Autodesk Inventor part; units mm, degrees
ref_plane "YZ Plane" through (0, 0, 0) normal (1, 0, 0) x (0, 1, 0)
ref_plane "XZ Plane" through (0, 0, 0) normal (0, 1, 0) x (-1, 0, 0)
ref_plane "XY Plane" through (0, 0, 0) normal (0, 0, 1) x (1, 0, 0)
sketch "Sketch1" plane through (0, 0, 0) normal (0, 1, 0) x (-1, 0, 0)
  line L0 (0, 0) -> (56, 0)
  line L1 (56, 0) -> (54.5, 0)
  line L2 (56, 0) -> (21.359, -20)
  line L3 (56, 0) -> (96, 0) construction
  line L4 (28, 0) -> (28, 5.9969)
  line L5 (0, 0) -> (34.641, -20)
  line L6 (28, 0) -> (28, -6)
  line L7 (28, -6) -> (78, -6)
  line L8 (28, -6) -> (-22, -6)
  line L9 (56, 0) -> (53.4019, -1.5)
  line L10 (53.4019, -1.5) -> (39.2598, -15.6421)
  line L11 (53.4019, -1.5) -> (73.4019, -1.5) construction
  line L12 (2.5981, -1.5) -> (16.7402, -15.6421)
  point P0 (48.9019, -6)
  point P1 (7.0981, -6)
  dimension "d0" = 56
  dimension "d3" = 40
  dimension "d4" = 150
  dimension "d5" = 6
  dimension "d6" = 50
  dimension "d7" = 50
  dimension "d8" = 3
  dimension "d9" = 20
  dimension "d10" = 135
extrude "Extrusion1" add sketch "Sketch1" along normal blind 6 contours L0 L6 L8 L5 | L0 L2 L7 L6 | L5 L8 L12 | L2 L10 L7
chamfer "Chamfer1" distance 2 angle 45 6 edges at (-48.9019, 3, -6) (-51.1519, 6, -3.75) (-51.1519, 0, -3.75) (-4.8481, 0, -3.75) (-7.0981, 3, -6) (-4.8481, 6, -3.75)
chamfer "Chamfer2" distance 2 angle 45 2 edges at (-37.0367, 0, -6) (-37.0367, 6, -6)
sketch "Sketch3" plane through (0, 0, 0) normal (0, -1, 0) x (1, 0, 0)
  line L0 (-49.0718, -4) -> (-56, 0)
  line L1 (-56, 0) -> (-32.5, 0)
  line L2 (-56, 0) -> (0, 0)
  line L3 (-32.5, 0) -> (-32.5, -2.5)
  line L4 (-6.9282, -4) -> (-49.0718, -4)
  circle A0 centre (-32.5, -2.5) radius 1.1
  dimension "d25" = 23.5
  dimension "d26" = 2.5
  dimension "d27" = 2.2
extrude "Extrusion3" cut sketch "Sketch3" against normal blind 50
properties part number "parallel_bar_long_hole_v1"
Check sheet for the modelled part. Datum: model origin and axes. Units: mm. A direction names the side the tool comes from. Round coordinates to 2 decimals unless told otherwise and drop trailing zeros. Loops run counter-clockwise (first coordinate to the right, second up) from the corner with the lowest first, then second, coordinate; pieces in that order, holes last. Notation, with made-up numbers: (27.5, 13.5) - (56.5, 13.5) arc R31 ccw to (56.5, 40.5) - close; hole circle Ø1 at (83, -23.75). An arc over 180 degrees is marked (long way). Write item = value, one per line. Start each with the question number.
Q1. Depth check by flat-ended pin: P1, Ø3, axis at y = 2, z = -5, coming from the +X side; P2, Ø1.3, axis at x = -32.5, z = -2.5, coming from the -Y side; P3, Ø1, axis at y = 1, z = -3, coming from the +X side. Enter the tip coordinate at first touch or a pass-through.
Q2. Release check for a two-part mould opening along X. For faces 1 (the face through (-28, 0, -2)), 2 (the face through (-31.45, 2.96, -2.17)), 3 (the face through (-2.094, 2.958, -1.209)) record: pulls with the +X half, pulls with the -X half, needs draft (parallel to the pull), parting line crosses it, or undercut.
Q3. Access from +Z, -Z, +X, -X, +Y, -Y to the whole of each face (thin tool, end or side, straight path). Record for faces 4 (the face through (-53.906, 2.958, -1.209)), 5 (the face through (-28, 3, 0)).
Q4. Thickness scan on L1, parallel to Z at x = -32.5, y = 2.75; L2, parallel to Z at x = -32.5, y = 1.3; L3, parallel to X at y = 4, z = -3.25. Record the ranges inside material, lowest first.
Q5. Section check D-D (x = -13.5). Record the boundary of the cut face in (y, z).
Q6. Section check B-B (z = -2.5). Record the boundary of the cut face in (x, y).
Q7. Section check A-A (x = -32.5). Record the boundary of the cut face in (y, z), plus the area to 3 significant figures.
Q8. Section check C-C (y = 3.25). Record the boundary of the cut face in (x, z).
Derived:
q1.P1 = -4.6
q1.P2 = through
q1.P3 = -4.33
q2.face_1 = needs draft
q2.face_2 = undercut
q2.face_3 = pulls with the +X half
q3.face_4 = -Z, -X
q3.face_5 = +Z, +X, -X, +Y, -Y
q4.L1 = -6 to -3.6, -1.4 to 0
q4.L2 = -5.3 to -3.6, -1.4 to 0
q4.L3 = -51.65 to -33.3, -31.7 to -4.35
q5.outline = (0, -4) - (2, -6) - (4, -6) - (6, -4) - (6, 0) - (0, 0) - close
q6.outline = (-52.4, 2) - (-51.67, 1.48) - (-51.67, 0) - (-33.6, 0) - (-33.6, 6) - (-51.67, 6) - (-51.67, 4.52) - (-52.4, 4) - close; (-31.4, 0) - (-4.33, 0) - (-4.33, 1.48) - (-3.6, 2) - (-3.6, 4) - (-4.33, 4.52) - (-4.33, 6) - (-31.4, 6) - close
q7.outline = (0, -4) - (2, -6) - (4, -6) - (6, -4) - (6, -3.6) - (0, -3.6) - close; (0, -1.4) - (6, -1.4) - (6, 0) - (0, 0) - close
q7.area = 18.8 mm^2
q8.outline = (-56, 0) - (-53.4, -1.5) - (-50.32, -4.59) - (-46.9, -6) - (-9.1, -6) - (-5.68, -4.59) - (-2.6, -1.5) - (0, 0) - close; hole circle Ø2.2 at (-32.5, -2.5)
